```python
from build123d import *

# Parameters (mm, degrees)
SKETCH1_W           = 152.4
SKETCH1_H           = 152.4
SKETCH1_R           = 59.69
BOSS_EXTRUDE1_DEPTH = 0.4191
SKETCH2_R           = 3.4925
SKETCH2_R_2         = 1.27
CUT_EXTRUDE1_DEPTH  = 108.766333236
CIRPATTERN1_COUNT   = 4


with BuildPart() as part:
    # Sketch1 → Boss-Extrude1 (new, symmetric)
    with BuildSketch(Plane(origin=(0, 0, 0), x_dir=(1, 0, 0), z_dir=(0, 1, 0))):
        Rectangle(SKETCH1_W, SKETCH1_H)
        with Locations(Location((0, 0, 0), (0, 0, 270))):
            Circle(SKETCH1_R, mode=Mode.SUBTRACT)
    extrude(amount=BOSS_EXTRUDE1_DEPTH, both=True)

    # Sketch2 → Cut-Extrude1 (cut, through all)
    with BuildSketch(Plane(origin=(0, 0.4191, 0), x_dir=(1, 0, 0), z_dir=(0, 1, 0))):
        with Locations(Location((-69.85, 69.85, 0), (0, 0, 270))):
            Circle(SKETCH2_R)
        with Locations(Location((-58.647249233, 69.85, 0), (0, 0, 270))):
            Circle(SKETCH2_R_2)
    cut_extrude1 = extrude(amount=-CUT_EXTRUDE1_DEPTH, mode=Mode.SUBTRACT)

    # CirPattern1: Cut-Extrude1 ×4 about axis
    cirpattern1_axis = Axis((0, 0, 0), (0, 1, 0))
    for i in range(1, CIRPATTERN1_COUNT):
        add(cut_extrude1.rotate(cirpattern1_axis, i * 360 / CIRPATTERN1_COUNT), mode=Mode.SUBTRACT)


solid = part.part
```
Geometry check sheet. Reference: the model listing, model coordinates, mm. Coordinates: 2 decimals unless noted, no trailing zeros. Order: outer loops, then holes, each group sorted by start corner. A loop starts at its lowest first (then second) coordinate and runs counter-clockwise, first axis right, second up. Notation, with made-up numbers: (52, 84) - (88, 84) arc R28 cw to (88, 122) - close; hole circle Ø9 at (3, 38). An arc over 180 degrees is marked (long way). Answer in a Markdown table with one row per item. Add a question column.
1. Section check B-B (x = -44.5). Enter the section's corners in (y, z).
2. Draft check along X on faces 1 (the face through (-66.905, 0.006, -67.972)), 2 (the face through (70.305, 0.006, -66.387)), 3 (the face through (-52, -0.419, -35)). Enter one of: +X half, -X half, draft (parallel to the pull), parting line (faces both ways), or undercut.
3. Section check C-C (y = -0.05). Give the number of separate pieces and of enclosed holes in the cut face, plus the area to 3 significant figures.
4. Material ranges on L1, parallel to X at y = 0, z = 69.85; L2, parallel to Z at x = 69.85, y = 0.25; L3, parallel to X at y = 0.05, z = 0, recorded low to high. Write a range as [from, to].
5. Gauge pin test, flat end, axial feed: pin 1 Ø8 at (x, z) = (50.5, 17.5) entering from -Y. Record the tip position at first contact, or that the pin passes through.
6. Section check A-A (z = 0). Enter the section's corners in (x, y).
Data:
| question | item | result |
|---|---|---|
| 1 | outline | (-0.42, -76.2) - (0.42, -76.2) - (0.42, -39.78) - (-0.42, -39.78) - close; (-0.42, 39.78) - (0.42, 39.78) - (0.42, 76.2) - (-0.42, 76.2) - close |
| 2 | face 1 | undercut |
| 2 | face 2 | undercut |
| 2 | face 3 | draft |
| 3 | separate pieces | 1 |
| 3 | enclosed holes | 9 |
| 3 | area | 11,900 mm² |
| 4 | L1 | x = [-76.2, -73.34], [-66.36, 57.38], [59.92, 66.36], [73.34, 76.2] |
| 4 | L2 | z = [-76.2, -73.34], [-66.36, -59.92], [-57.38, 66.36], [73.34, 76.2] |
| 4 | L3 | x = [-76.2, -59.69], [59.69, 76.2] |
| 5 | pin 1 | passes through |
| 6 | outline | (-76.2, -0.42) - (-59.69, -0.42) - (-59.69, 0.42) - (-76.2, 0.42) - close; (59.69, -0.42) - (76.2, -0.42) - (76.2, 0.42) - (59.69, 0.42) - close |
